Here's how the part is built. I have some questions about the finished solid (model axes, mm). Face numbers are marked on the shaded views. A direction names the side the tool comes from. Give positions to 0.01 mm unless a question says otherwise; leave off trailing zeros. Write each loop counter-clockwise with the first axis right and the second up, starting at its lowest first coordinate (ties: lowest second). Pieces come first, ordered by that corner, then holes. Notation, with made-up numbers: (-29.5, -6.5) -> (-11.5, -6.5) arc R19 ccw to (-11.5, 10.5) -> close; hole circle Ø5 at (42.5, 71.5). An arc over 180 degrees is marked (long way). Use CSV: the item, a comma, the result in double quotes. Start each with the question number.
(1) Which directions (+Z, -Z, +X, -X, +Y, -Y) give clear straight access to the entire face, cutting with the end or side of a thin tool? Please do the marked faces 5, 6, 7 and 8.
(2) I need wall thicknesses on L1, parallel to Y at x = 0, z = 2.85; L2, parallel to Y at x = -6, z = 1.8; L3, parallel to X at y = -8, z = 3.85. Which ranges of each line are inside material? Lowest first, please. Write a range as [from, to].
(3) For pin 1 Ø1.6 at (y, z) = (-15, 4.5) entering from +X; pin 2 Ø2 at (y, z) = (15, 2.5) entering from -X; pin 3 Ø1 at (x, z) = (15, 3) entering from -Y, each with a flat end and sliding along its axis, tell me the tip position at first contact or that it passes through.
(4) Suppose I cut it at C-C on z = 4.4. List the corners of the cut face in (x, y) for me.
(5) If we mould it in two halves opening along X, with no side actions, what happens to the marked faces 1, 2, 3 and 4? For each: pulls with the +X half, pulls with the -X half, needs draft (parallel to the pull), parting line crosses it, or undercut.
(6) Suppose I cut it at A-A on x = 0. List the corners of the cut face in (y, z) for me, plus the area to 3 significant figures.
from build123d import *

# Parameters (mm, degrees)
ESQUISSE2_OUTSIDE_W     = 43.13
ESQUISSE2_OUTSIDE_H     = 43.13
ENL_V_MAT_EXTRU_2_DEPTH = 24.409399821


with BuildPart() as part:
    # Esquisse1 → Base-Révolution (revolve)
    with BuildSketch(Plane(origin=(0, 0, 0), x_dir=(0, 0, -1), z_dir=(1, 0, 0)), mode=Mode.PRIVATE) as base_r_volution_sk:
        Polygon((0, 10), (0, 13), (-1.732050808, 16), (-6, 16), (-6, 10), align=None)
    revolve(base_r_volution_sk.sketch.rotate(Axis((0, 0, 0), (0, 0, 1)), 90), axis=Axis((0, 0, 0), (0, 0, 1)))

    # Esquisse2 outside → Enlèv. mat.-Extru.2 (cut, through all)
    with BuildSketch(Plane.XY):
        Rectangle(ESQUISSE2_OUTSIDE_W, ESQUISSE2_OUTSIDE_H)
        with BuildLine():
            Line((-2, 13.874507866), (2, 13.874507866))
            Line((2, 13.874507866), (2, 15.874507866))
            ThreePointArc((2, 15.874507866), (11.313708499, 11.313708499), (15.874507866, 2))
            Line((15.874507866, 2), (13.874507866, 2))
            Line((13.874507866, 2), (13.874507866, -2))
            Line((13.874507866, -2), (15.874507866, -2))
            ThreePointArc((15.874507866, -2), (11.313708499, -11.313708499), (2, -15.874507866))
            Line((2, -15.874507866), (2, -13.874507866))
            Line((2, -13.874507866), (-2, -13.874507866))
            Line((-2, -13.874507866), (-2, -15.874507866))
            ThreePointArc((-2, -15.874507866), (-11.313708499, -11.313708499), (-15.874507866, -2))
            Line((-15.874507866, -2), (-13.874507866, -2))
            Line((-13.874507866, -2), (-13.874507866, 2))
            Line((-13.874507866, 2), (-15.874507866, 2))
            ThreePointArc((-15.874507866, 2), (-11.313708499, 11.313708499), (-2, 15.874507866))
            Line((-2, 15.874507866), (-2, 13.874507866))
        make_face(mode=Mode.SUBTRACT)
    extrude(amount=ENL_V_MAT_EXTRU_2_DEPTH, mode=Mode.SUBTRACT)


solid = part.part
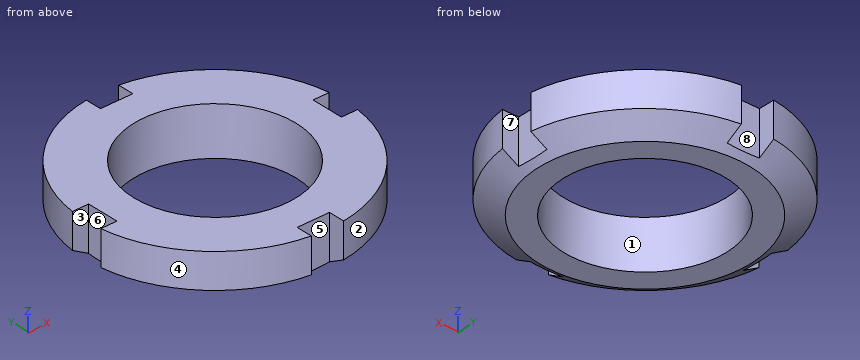
Geometry says:
1,face 5,"+Z, -Z, -Y"
1,face 6,"+Z, -Z, -X"
1,face 7,"+Z, -Z, +X"
1,face 8,"+Z, -Z, +Y"
2,L1,"[-13.87, -10], [10, 13.87]"
2,L2,"[-14.83, -8], [8, 14.83]"
2,L3,"[-13.86, -6], [6, 13.86]"
3,pin 1,"x = 7.37"
3,pin 2,"x = -7.75"
3,pin 3,"y = -6.76"
4,outline,"(-15.87, -2) arc R16 ccw to (-2, -15.87) -> (-2, -13.87) -> (2, -13.87) -> (2, -15.87) arc R16 ccw to (15.87, -2) -> (13.87, -2) -> (13.87, 2) -> (15.87, 2) arc R16 ccw to (2, 15.87) -> (2, 13.87) -> (-2, 13.87) -> (-2, 15.87) arc R16 ccw to (-15.87, 2) -> (-13.87, 2) -> (-13.87, -2) -> close; hole circle Ø20 at (0, 0)"
5,face 1,"undercut"
5,face 2,"pulls with the +X half"
5,face 3,"needs draft"
5,face 4,"pulls with the -X half"
6,outline,"(-13.87, 0.5) -> (-13, 0) -> (-10, 0) -> (-10, 6) -> (-13.87, 6) -> close; (10, 0) -> (13, 0) -> (13.87, 0.5) -> (13.87, 6) -> (10, 6) -> close"
6,area,"46.1 mm²"
